Geometry check sheet. Reference: the model listing, model coordinates, mm. Face numbers are marked on the shaded views. A direction names the side the tool comes from. Round coordinates to 2 decimals unless told otherwise and drop trailing zeros. Write each loop counter-clockwise with the first axis right and the second up, starting at its lowest first coordinate (ties: lowest second). Pieces come first, ordered by that corner, then holes.
Item 1: Draft check along X on the marked faces 1 and 2. Enter one of: pulls with the +X half, pulls with the -X half, needs draft (parallel to the pull), parting line crosses it, or undercut.
Item 2: Cross-section at D-D (z = -11.5). Enter the section's corners in (x, y), then the cut area to 3 significant figures.
Item 3: Depth check by flat-ended pin: P1, Ø3, axis at y = 10, z = 0, coming from the -X side; P2, Ø4, axis at x = 17, z = 5, coming from the -Y side; P3, Ø8, axis at x = 33, z = 13.5, coming from the +Y side; P4, Ø5, axis at x = 45, y = 10.5, coming from the -Z side. Enter the tip coordinate at first touch or a pass-through.
Item 4: Scan lines: probe 1 along X at (y, z) = (9, 1); probe 2 along Y at (x, z) = (-45, 0); probe 3 along Z at (x, y) = (-46.5, 10). Record each from-to range of solid material in increasing order.
Item 5: Cross-section at C-C (x = -31.5). Enter the section's corners in (y, z), then the cut area to 3 significant figures.
Item 6: Cross-section at B-B (y = 10). Enter the section's corners in (x, z), then the cut area to 3 significant figures.
Item 7: Cross-section at A-A (z = 0). Enter the section's corners in (x, y), then the cut area to 3 significant figures.
Item 8: Access from +Z, -Z, +X, -X, +Y, -Y to the whole of each face (thin tool, end or side, straight path). Record for the marked faces 3 and 4.
from build123d import *

# Parameters (mm, degrees)
EXTRUDE_1_DEPTH     = 3
EXTRUDE_2_DEPTH     = 5
SKETCH_4_R          = 1
CUT_EXTRUDE_1_DEPTH = 101
EXTRUDE_3_DEPTH     = 3


with BuildPart() as part:
    # Эскиз1 → Бобышка-Вытянуть1 (new body)
    with BuildSketch(Plane(origin=(0, 0, 0), x_dir=(1, 0, 0), z_dir=(0, 1, 0))):
        with BuildLine():
            Line((-45, -21.5), (45, -21.5))
            ThreePointArc((45, -21.5), (48.535533906, -20.035533906), (50, -16.5))
            Line((50, -16.5), (50, 16.5))
            ThreePointArc((50, 16.5), (48.535533906, 20.035533906), (45, 21.5))
            Line((45, 21.5), (-45, 21.5))
            ThreePointArc((-45, 21.5), (-48.535533906, 20.035533906), (-50, 16.5))
            Line((-50, 16.5), (-50, -16.5))
            ThreePointArc((-50, -16.5), (-48.535533906, -20.035533906), (-45, -21.5))
        make_face()
    extrude(amount=EXTRUDE_1_DEPTH)

    # Эскиз3 → Бобышка-Вытянуть2 (add, symmetric)
    with BuildSketch(Plane.XY):
        Polygon((-39.226497308, 3), (-45, 3), (-50, 3), (-50, 13), (-45, 13), align=None)
        Polygon((50, 3), (45, 3), (39.226497308, 3), (45, 13), (50, 13), align=None)
    extrude(amount=EXTRUDE_2_DEPTH, both=True)

    # Эскиз4 → Вырез-Вытянуть1 (cut, through all)
    with BuildSketch(Plane.ZY.offset(50)):
        with Locations((0, 10)):
            Circle(SKETCH_4_R)
    extrude(amount=-CUT_EXTRUDE_1_DEPTH, mode=Mode.SUBTRACT)

    # Эскиз5 → Бобышка-Вытянуть3 (add)
    with BuildSketch(Plane.XZ):
        with BuildLine():
            Line((52, -18.5), (52, -16.5))
            Line((52, -16.5), (52, 16.5))
            Line((52, 16.5), (52, 18.5))
            ThreePointArc((52, 18.5), (50.535533906, 22.035533906), (47, 23.5))
            Line((47, 23.5), (45, 23.5))
            Line((45, 23.5), (-45, 23.5))
            Line((-45, 23.5), (-47, 23.5))
            ThreePointArc((-47, 23.5), (-50.535533906, 22.035533906), (-52, 18.5))
            Line((-52, 18.5), (-52, 16.5))
            Line((-52, 16.5), (-52, -16.5))
            Line((-52, -16.5), (-52, -18.5))
            ThreePointArc((-52, -18.5), (-50.535533906, -22.035533906), (-47, -23.5))
            Line((-47, -23.5), (-45, -23.5))
            Line((-45, -23.5), (45, -23.5))
            Line((45, -23.5), (47, -23.5))
            ThreePointArc((47, -23.5), (50.535533906, -22.035533906), (52, -18.5))
        make_face()
        with BuildLine():
            Line((50, 16.5), (50, -16.5))
            ThreePointArc((50, -16.5), (48.535533906, -20.035533906), (45, -21.5))
            Line((45, -21.5), (-45, -21.5))
            ThreePointArc((-45, -21.5), (-48.535533906, -20.035533906), (-50, -16.5))
            Line((-50, -16.5), (-50, 16.5))
            ThreePointArc((-50, 16.5), (-48.535533906, 20.035533906), (-45, 21.5))
            Line((-45, 21.5), (45, 21.5))
            ThreePointArc((45, 21.5), (48.535533906, 20.035533906), (50, 16.5))
        make_face(mode=Mode.SUBTRACT)
    extrude(amount=-EXTRUDE_3_DEPTH)


solid = part.part
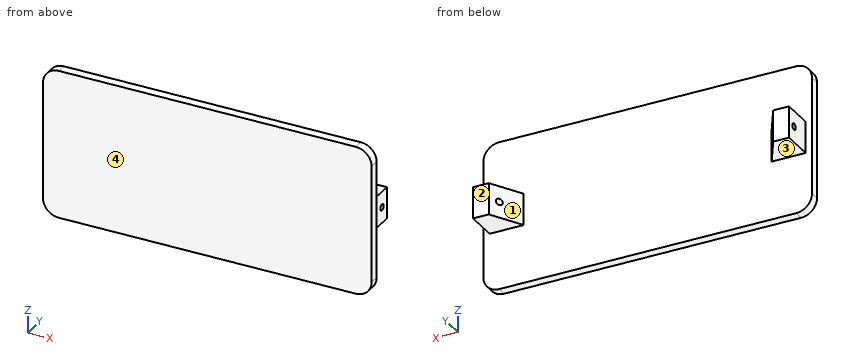
Resolved:
1. face 1: undercut
1. face 2: needs draft
2. outline: (-52, 0) - (52, 0) - (52, 3) - (-52, 3) - close
2. area: 312 mm2
3. P1: stops at x = -50
3. P2: stops at y = 0
3. P3: stops at y = 3
3. P4: stops at z = -5
4. probe 1: x = -50 to -42.69, 42.69 to 50
4. probe 2: y = 0 to 9, 11 to 13
4. probe 3: z = -5 to -1, 1 to 5
5. outline: (0, -23.5) - (3, -23.5) - (3, 23.5) - (0, 23.5) - close
5. area: 141 mm2
6. outline: (-50, -5) - (-43.27, -5) - (-43.27, -1) - (-50, -1) - close; (-50, 1) - (-43.27, 1) - (-43.27, 5) - (-50, 5) - close; (43.27, -5) - (50, -5) - (50, -1) - (43.27, -1) - close; (43.27, 1) - (50, 1) - (50, 5) - (43.27, 5) - close
6. area: 108 mm2
7. outline: (-52, 0) - (52, 0) - (52, 3) - (50, 3) - (50, 9) - (42.69, 9) - (39.23, 3) - (-39.23, 3) - (-42.69, 9) - (-50, 9) - (-50, 3) - (-52, 3) - close; (-50, 11) - (-43.85, 11) - (-45, 13) - (-50, 13) - close; (43.85, 11) - (50, 11) - (50, 13) - (45, 13) - close
7. area: 443 mm2
8. face 3: -Z, +X, -X, +Y
8. face 4: +Z, -Z, +X, -X, -Y
